Geometry: final body of the model. Coordinates: model frame, mm. Face numbers are marked on the shaded views. Give positions to 0.01 mm unless a question says otherwise; leave off trailing zeros. Write each loop counter-clockwise with the first axis right and the second up, starting at its lowest first coordinate (ties: lowest second). Pieces come first, ordered by that corner, then holes. Notation, with made-up numbers: M -12.5,59 L 31.5,59 A29 cw 31.5,98 Z; hole C 73.25,22 d11. An arc over 180 degrees is marked long. Use one line per item in the form item = value. Start each with the question number.
Item 1: Section query D-D on x = 18.5. Return loops of the section in (y, z).
Item 2: Section query A-A on z = -35. Return loops of the section in (x, y), then the cut area to 3 significant figures.
Item 3: Section query C-C on y = -4. Return loops of the section in (x, z).
Item 4: Material intervals for line 1 along X through (y, z) = (-4.95, -34); line 2 along Z through (x, y) = (0, -4.7); line 3 along Z through (x, y) = (12, -0.75), sorted ascending. Write a range as from..to.
Item 5: Section query B-B on x = 12. Return loops of the section in (y, z).
Item 6: Pull-direction query (X, two-part tool) for the marked faces 1, 2 and 3; classes: released by +X, released by -X, zero draft, split by the parting line, or undercut.
Item 7: Contact query for flat-ended pins moving along their axis: P1, Ø7, axis at x = -12, z = -35, coming from the -Y side; P2, Ø9, axis at x = 12, z = -35, coming from the -Y side; P3, Ø2, axis at x = 8.5, y = -0.5, coming from the +Z side. Output: stop coordinate, or through.
from build123d import *

# Parameters (mm, degrees)
F0_R     = 2.75
F1_DEPTH = 6
F2_R     = 1
F3_SIZE  = 3


with BuildPart() as f1:
    # F0 (on Front) → F1 (new body)
    with BuildSketch(Plane.XZ):
        with BuildLine():
            ThreePointArc((21, 0), (0, -21), (-21, 0))
            Line((-21, 0), (-21, -40))
            ThreePointArc((-21, -40), (-18.071068, -47.071068), (-11, -50))
            Line((-11, -50), (11, -50))
            ThreePointArc((11, -50), (18.071068, -47.071068), (21, -40))
            Line((21, -40), (21, 0))
        make_face()
        with Locations((-12, -35)):
            Circle(F0_R, mode=Mode.SUBTRACT)
        with Locations((12, -35)):
            Circle(F0_R, mode=Mode.SUBTRACT)
    extrude(amount=F1_DEPTH)

    # F2
    f2_edges = [f1.edges().sort_by_distance(p)[0] for p in [
        (-21, -3, 0),
        (21, -3, 0),
    ]]
    fillet(f2_edges, radius=F2_R)

    # F3
    f3_edges = [f1.edges().sort_by_distance(p)[0] for p in [
        (-14.75, -6, -35),
        (9.25, -6, -35),
    ]]
    chamfer(f3_edges, length=F3_SIZE)


solid = f1.part
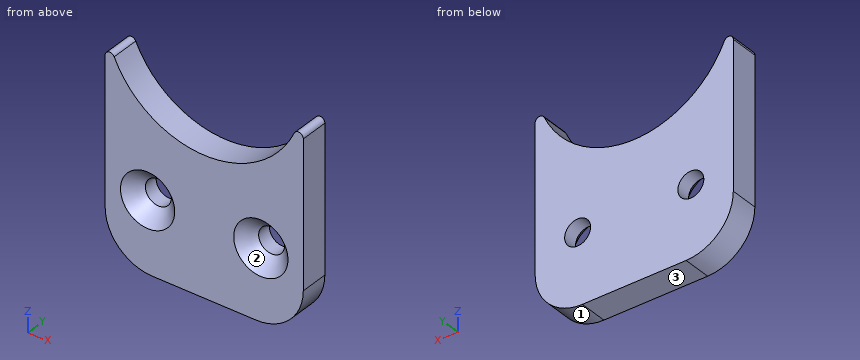
Answer sheet:
q1.outline = M -6,-46.61 L 0,-46.61 L 0,-9.94 L -6,-9.94 Z
q2.outline = M -21,-6 L -17.75,-6 L -14.75,-3 L -14.75,0 L -21,0 Z; M -9.25,-3 L -6.25,-6 L 6.25,-6 L 9.25,-3 L 9.25,0 L -9.25,0 Z; M 14.75,-3 L 17.75,-6 L 21,-6 L 21,0 L 14.75,0 Z
q2.area = 168 mm2
q3.outline = M -21,-40 A10 ccw -11,-50 L 11,-50 A10 ccw 21,-40 L 21,-9.17 A1 ccw 19.09,-8.75 A21 cw -19.09,-8.75 A1 ccw -21,-9.17 Z; hole C -12,-35 d7.5; hole C 12,-35 d7.5
q4.line_1 = -21..-16.59, -7.41..7.41, 16.59..21
q4.line_2 = -50..-21
q4.line_3 = -49.95..-37.75, -32.25..-17.23
q5.outline = M -6,-49.95 L 0,-49.95 L 0,-37.75 L -3,-37.75 L -6,-40.75 Z; M -6,-29.25 L -3,-32.25 L 0,-32.25 L 0,-17.23 L -6,-17.23 Z
q6.face_1 = released by +X
q6.face_2 = undercut
q6.face_3 = zero draft
q7.P1 = -3.75
q7.P2 = -4.75
q7.P3 = -18.73
